Model file for the job. Use its own axes, mm. Face numbers are marked on the shaded views. Coordinates: 2 decimals unless noted, no trailing zeros. Write each loop counter-clockwise with the first axis right and the second up, starting at its lowest first coordinate (ties: lowest second). Pieces come first, ordered by that corner, then holes. Notation, with made-up numbers: (-16.75, 73.5) -> (32.25, 73.5) arc R22 ccw to (32.25, 104.5) -> close; hole circle Ø7 at (47, 56.5). An arc over 180 degrees is marked (long way). Answer as a JSON object with one key per item and string values. Group by question number.
Solid Edge part; units mm, degrees
sketch "Sketch1" plane through (0, 0, 0) normal (0, 0, 1) x (1, 0, 0)
  line L0 (-56.1534, -25.9068) -> (57.8466, -25.9068)
  line L1 (57.8466, -25.9068) -> (57.8466, 40.0932)
  line L2 (57.8466, 40.0932) -> (-56.1534, 40.0932)
  line L3 (-56.1534, 40.0932) -> (-56.1534, -25.9068)
extrude "Protrusion1" add sketch "Sketch1" along normal blind 2
sketch "Sketch2" plane through (0.8466, 7.0932, 2) normal (0, 0, 1) x (1, 0, 0)
  line L0 (-55, 31) -> (-55, -31)
  line L1 (-55, -31) -> (55, -31)
  line L2 (55, -31) -> (55, 31)
  line L3 (55, 31) -> (-55, 31)
extrude "ExtrudedProtrusion_2" add sketch "Sketch2" along normal blind 2
sketch "Sketch3" plane through (0.8466, 7.0932, 4) normal (0, 0, 1) x (1, 0, 0)
  line L0 (-53, 29) -> (-53, -29)
  line L1 (-53, -29) -> (53, -29)
  line L2 (53, -29) -> (53, 27)
  line L3 (53, 27) -> (53, 29)
  line L4 (53, 29) -> (-53, 29)
extrude "ExtrudedCutout_1" cut sketch "Sketch3" against normal blind 2
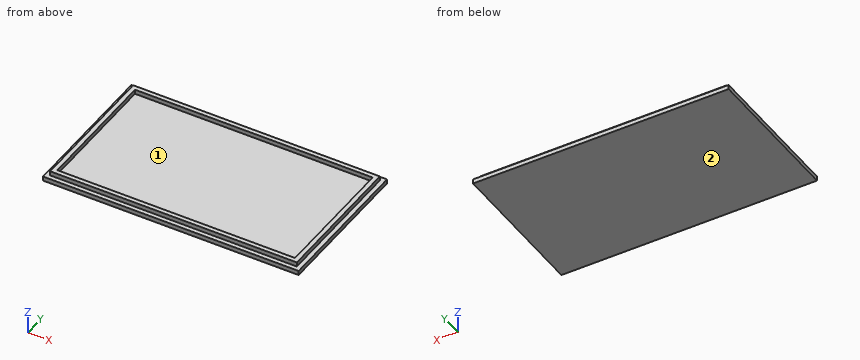
(1) Wall check: probe 1 along X at (y, z) = (-9, 3.1); probe 2 along Y at (x, z) = (-44.5, 2.05); probe 3 along Z at (x, y) = (-9, -6). Give the ranges that are in metal, low to high.
(2) Pull direction Y, two halves, no side cores. Call the marked faces 1 and 2: released by +Y, released by -Y, zero draft, split by the parting line, or undercut.
(3) Pin check, flat tips, straight feed: pin 1 (1 mm diameter, centred on y = 13, z = 3.5, fed in from -X); pin 2 (1.6 mm diameter, centred on y = 6.5, z = 3.5, fed in from +X); pin 3 (1 mm diameter, centred on x = 9.5, z = 3, fed in from +Y). Stop position of each tip, or through.
(4) Cut at A-A on x = 21. List the corners of the cut face in (y, z), plus the area to 3 significant figures.
(5) Cut at B-B on y = 11.5. List the corners of the cut face in (x, z), plus the area to 3 significant figures.
Results found:
{
 "1": {"probe 1": "x = -54.15 to -52.15, 53.85 to 55.85", "probe 2": "y = -23.91 to -21.91, 36.09 to 38.09", "probe 3": "z = 0 to 2"},
 "2": {"face 1": "undercut", "face 2": "zero draft"},
 "3": {"pin 1": "stops at x = -54.15", "pin 2": "stops at x = 55.85", "pin 3": "stops at y = 38.09"},
 "4": {"outline": "(-25.91, 0) -> (40.09, 0) -> (40.09, 2) -> (38.09, 2) -> (38.09, 4) -> (36.09, 4) -> (36.09, 2) -> (-21.91, 2) -> (-21.91, 4) -> (-23.91, 4) -> (-23.91, 2) -> (-25.91, 2) -> close", "area": "140 mm²"},
 "5": {"outline": "(-56.15, 0) -> (57.85, 0) -> (57.85, 2) -> (55.85, 2) -> (55.85, 4) -> (53.85, 4) -> (53.85, 2) -> (-52.15, 2) -> (-52.15, 4) -> (-54.15, 4) -> (-54.15, 2) -> (-56.15, 2) -> close", "area": "236 mm²"}
}
